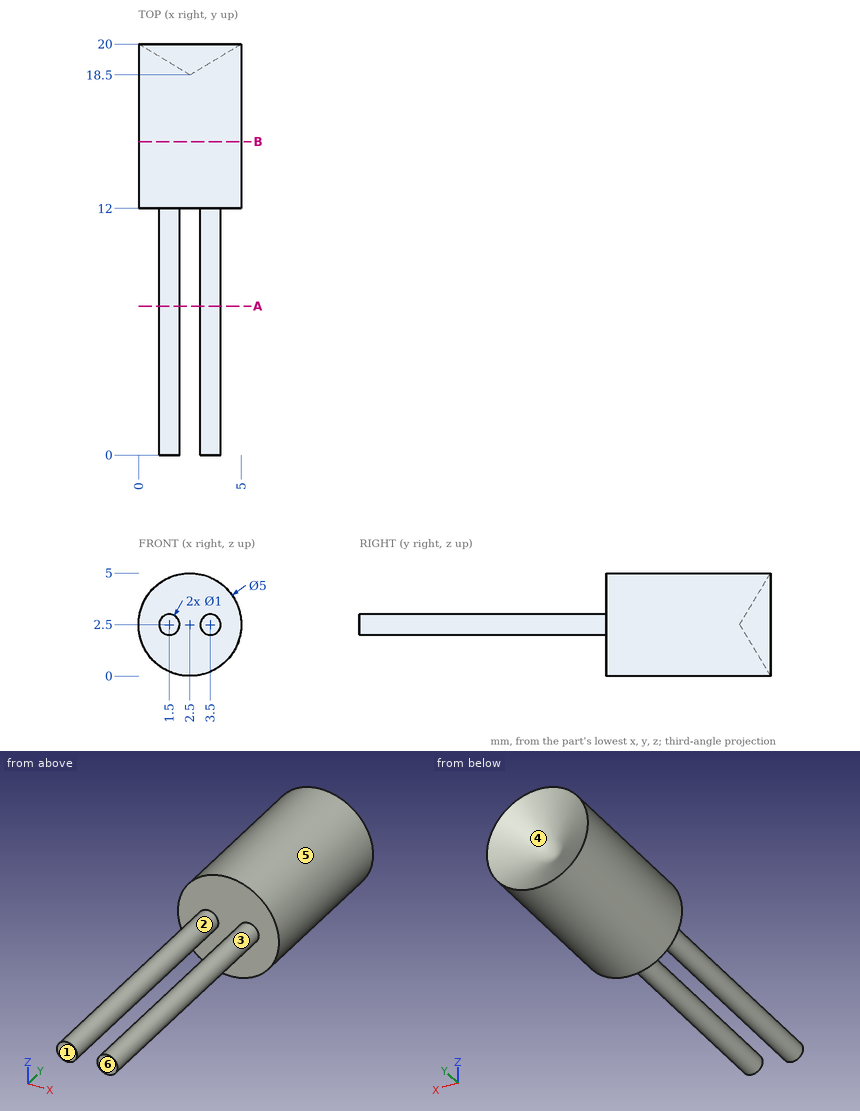
Part print with two shaded views. Sizes in mm from the minimum x, y, z corner. A direction names the side the tool comes from. Give positions to 0.01 mm unless a question says otherwise; leave off trailing zeros. Loops run counter-clockwise (first coordinate to the right, second up) from the corner with the lowest first, then second, coordinate; pieces in that order, holes last. Notation, with made-up numbers: (-0.5, 12) - (32.5, 12) arc R23 ccw to (32.5, 31) - close; hole circle Ø7 at (85.5, 36.5). An arc over 180 degrees is marked (long way). Put each result on its own line as item: value.
Q1. Flat gauge pins, fed straight in: pin 1 (2 mm diameter, centred on x = 3.5, y = 15, fed in from -Z); pin 2 (1 mm diameter, centred on x = 0.5, z = 4.5, fed in from -Y); pin 3 (3 mm diameter, centred on x = 2.5, z = 3, fed in from +Y); pin 4 (2 mm diameter, centred on x = 1.5, z = 1.5, fed in from +Y). Where does each tip first touch, or does it go through?
Filled in:
pin 1: stops at z = 0
pin 2: stops at y = 12
pin 3: stops at y = 19.7
pin 4: stops at y = 19.95
Q2. Tool access for the marked faces 1 and 2: list every direction of +Z, -Z, +X, -X, +Y, -Y with a clear straight run to the whole face (end or side of a thin tool).
Filled in:
face 1: +Z, -Z, +X, -X, -Y
face 2: -Y
Q3. Slice it at A-A (y = 7.25). Give the cut face in (x, z), plus the area to 3 significant figures.
Filled in:
outline: circle Ø1 at (1.5, 2.5); circle Ø1 at (3.5, 2.5)
area: 1.57 mm²
Q4. Mould opens along X. For the marked faces 3, 4, 5 and 6 say: pulls with the +X half, pulls with the -X half, needs draft (parallel to the pull), parting line crosses it, or undercut.
Filled in:
face 3: undercut
face 4: undercut
face 5: parting line crosses it
face 6: needs draft
Q5. Probe line 1 along X through (y, z) = (3, 2.55); line 2 along Y through (x, z) = (1.4, 1.25); line 3 along Y through (x, z) = (1.95, 4.45). List the from-to ranges inside material, lowest first.
Filled in:
line 1: x = 1 to 2, 3 to 4
line 2: y = 12 to 19.5
line 3: y = 12 to 19.72
Q6. Slice it at B-B (y = 15.25). Give the cut face in (x, z), plus the area to 3 significant figures.
Filled in:
outline: circle Ø5 at (2.5, 2.5)
area: 19.6 mm²
